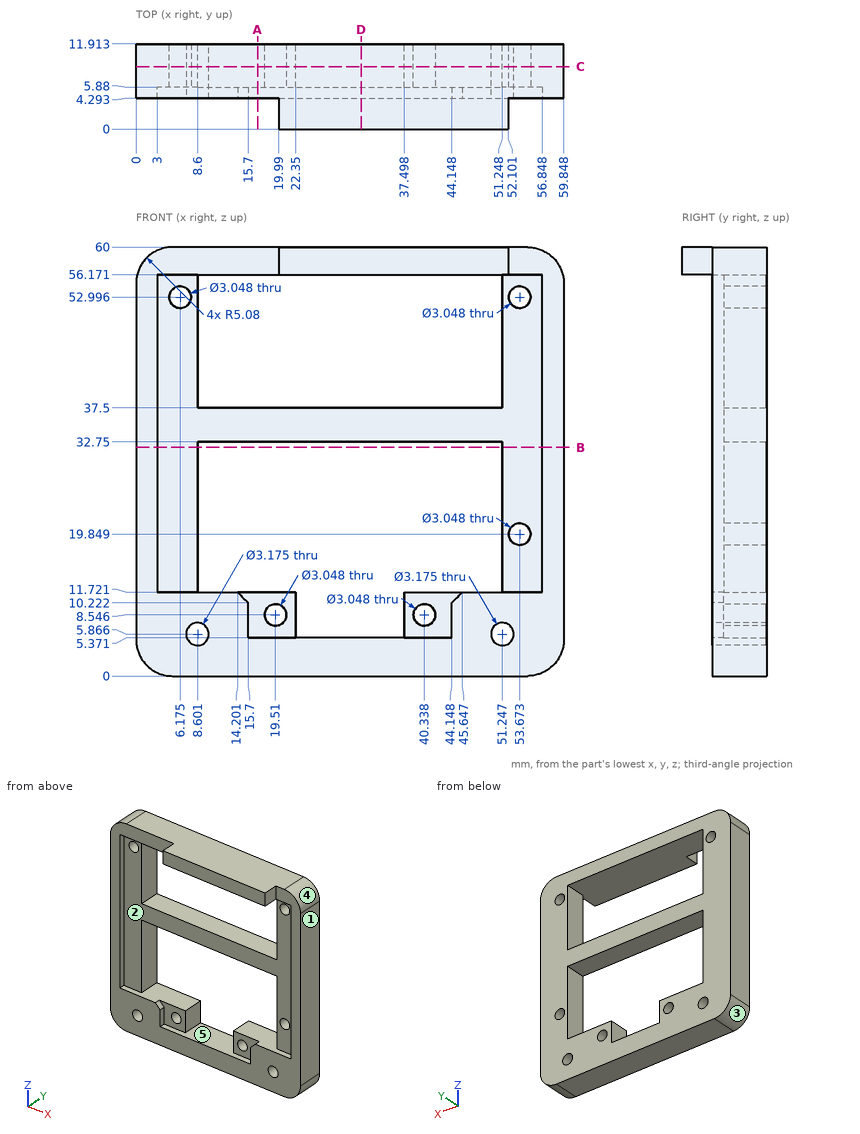
Geometry: see drawing. Coordinates: mm, zero at the bounding-box minimum. A direction names the side the tool comes from. Coordinates: 2 decimals unless noted, no trailing zeros. Loops run counter-clockwise (first coordinate to the right, second up) from the corner with the lowest first, then second, coordinate; pieces in that order, holes last. Notation, with made-up numbers: (71.5, 36.25) -> (77.5, 36.25) arc R14 cw to (77.5, 63.25) -> close; hole circle Ø11 at (16, 46.25). An arc over 180 degrees is marked (long way). Write item = value, one per line. Start each with the question number.
Item 1: Reachability of the marked faces 4 and 5 from +Z, -Z, +X, -X, +Y, -Y: full face, straight path, thin tool, end or side. Return the list, or none.
Item 2: Cut plane A-A, the plane x = 17. Return loops of the section in (y, z), plus the area to 3 significant figures.
Item 3: Cut plane C-C, the plane y = 8.75. Count the separate pieces of the cut face and the enclosed holes in it, plus the area to 3 significant figures.
Item 4: Cut plane D-D, the plane x = 31.5. Return loops of the section in (y, z).
Item 5: Cut plane B-B, the plane z = 32. Return loops of the section in (x, y).
Item 6: Mould query, pull axis Z, two halves, no side actions, for the marked faces 1, 2 and 3. Classes: pulls with the +Z half, pulls with the -Z half, needs draft (parallel to the pull), parting line crosses it, or undercut.
Item 7: Material intervals for line 1 (Z direction, x = 22.5, y = 11.75); line 2 (Z direction, x = 15.5, y = 9.25); line 3 (Z direction, x = 19.51, y = 9.5), sorted ascending.
Item 8: First-contact query: P1, Ø4, axis at x = 40.34, z = 8.55, coming from the -Y side. Flat tip, straight axial feed; report the tip coordinate or a pass-through.
Ans:
q1.face_4 = +Z, +X, +Y, -Y
q1.face_5 = -Y
q2.outline = (4.29, 0) -> (11.91, 0) -> (11.91, 11.72) -> (5.88, 11.72) -> (5.88, 5.37) -> (4.29, 5.37) -> close; (4.29, 56.17) -> (11.91, 56.17) -> (11.91, 60) -> (4.29, 60) -> close; (5.88, 32.75) -> (11.91, 32.75) -> (11.91, 37.5) -> (5.88, 37.5) -> close
q2.area = 137 mm²
q3.separate_pieces = 1
q3.enclosed_holes = 9
q3.area = 1,730 mm²
q4.outline = (0, 56.17) -> (11.91, 56.17) -> (11.91, 60) -> (0, 60) -> close; (4.29, 0) -> (11.91, 0) -> (11.91, 5.37) -> (4.29, 5.37) -> close; (5.88, 32.75) -> (11.91, 32.75) -> (11.91, 37.5) -> (5.88, 37.5) -> close
q5.outline = (0, 4.29) -> (3, 4.29) -> (3, 5.88) -> (8.6, 5.88) -> (8.6, 11.91) -> (0, 11.91) -> close; (51.25, 5.88) -> (56.85, 5.88) -> (56.85, 4.29) -> (59.85, 4.29) -> (59.85, 11.91) -> (51.25, 11.91) -> close
q6.face_1 = needs draft
q6.face_2 = undercut
q6.face_3 = pulls with the -Z half
q7.line_1 = 0 to 5.37, 32.75 to 37.5, 56.17 to 60
q7.line_2 = 0 to 11.72, 32.75 to 37.5, 56.17 to 60
q7.line_3 = 0 to 7.02, 10.07 to 11.72, 32.75 to 37.5, 56.17 to 60
q8.P1 = 5.88
